```python
from build123d import *

# Parameters (mm, degrees)
RESSALTO_EXTRUS_O1_DEPTH         = 5
ESBO_O2_W                        = 10
ESBO_O2_H                        = 30
ESBO_O2_W_2                      = 30
ESBO_O2_H_2                      = 8
CORTE_EXTRUS_O1_DEPTH            = 5
RESSALTO_EXTRUS_O2_DEPTH         = 5
FURO_COM_FOLGA_DE_M61_D          = 6.6
FURO_COM_FOLGA_DE_M51_D          = 5.5
CORTE_EXTRUS_O2_DEPTH            = 427.059799089
ESBO_O9_W                        = 4
ESBO_O9_H                        = 100
CORTE_EXTRUS_O3_DEPTH            = 417.461117513
FURO_COM_FOLGA_DE_M52_AT_2_COUNT = 2
FURO_COM_FOLGA_DE_M52_AT_2_PITCH = 36.977943225
FURO_COM_FOLGA_DE_M52_AT_3_COUNT = 2
FURO_COM_FOLGA_DE_M52_AT_3_PITCH = 73.955886449


with BuildPart() as part:
    # Esboço1 → Ressalto-extrusão1 (new body)
    with BuildSketch(Plane.XY):
        Polygon((230, 172.82), (360, 172.82), (360, 0), (0, 0), (0, 172.82), (130, 172.82), (130, 134.82), (230, 134.82), align=None)
    extrude(amount=RESSALTO_EXTRUS_O1_DEPTH)

    # Esboço2 → Corte-extrusão1 (cut)
    with BuildSketch(Plane.XY.offset(5)):
        with Locations((5, 61.5)):
            Rectangle(ESBO_O2_W, ESBO_O2_H)
        with Locations((355, 61.5)):
            Rectangle(ESBO_O2_W, ESBO_O2_H)
        with Locations((180, 4)):
            Rectangle(ESBO_O2_W_2, ESBO_O2_H_2)
    extrude(amount=-CORTE_EXTRUS_O1_DEPTH, mode=Mode.SUBTRACT)

    # Esboço3 → Ressalto-extrusão2 (add)
    with BuildSketch(Plane.XY.offset(5)):
        Polygon((360, 172.82), (360, 187.82), (250, 227.82), (250, 172.82), align=None)
        Polygon((0, 187.82), (110, 227.82), (110, 172.82), (0, 172.82), align=None)
    extrude(amount=-RESSALTO_EXTRUS_O2_DEPTH)

    # Furo com folga de M61 (through all)
    with Locations(Plane(origin=(0, 0, 0), x_dir=(-1, 0, 0), z_dir=(0, 0, -1))):
        with Locations((-355, 24.65), (-355, 86.5), (-5, 24.65), (-5, 86.5), (-320, 128.82), (-290, 128.82), (-70, 128.82), (-40, 128.82), (-177, 128.82), (-355, 101.5), (-5, 101.5), (-260, 128.82), (-100, 128.82), (-152, 128.82)):
            Hole(FURO_COM_FOLGA_DE_M61_D / 2)

    # Furo com folga de M51 (through all)
    with Locations(Plane(origin=(0, 0, 0), x_dir=(-1, 0, 0), z_dir=(0, 0, -1))):
        with Locations((-312, 17), (-312, 52.5), (-306.78, 4), (-207.78, 4), (-152.22, 4), (-53.22, 4)):
            furo_com_folga_de_m51 = Hole(FURO_COM_FOLGA_DE_M51_D / 2)

    # Espelhar1: Furo com folga de M51 across plane
    add(furo_com_folga_de_m51.mirror(Plane(origin=(180, 0, 0), x_dir=(0, 0, 1), z_dir=(1, 0, 0))), mode=Mode.SUBTRACT)

    # Esboço8 → Corte-extrusão2 (cut, through all)
    with BuildSketch(Plane.XY.offset(5)):
        Polygon((0, 187.82), (110, 227.82), (110, 209.32), (0, 171.82), align=None)
        Polygon((250, 209.32), (360, 171.82), (360, 187.82), (250, 227.82), align=None)
    extrude(amount=-CORTE_EXTRUS_O2_DEPTH, mode=Mode.SUBTRACT)

    # Esboço9 → Corte-extrusão3 (cut, through all)
    with BuildSketch(Plane.XY.offset(5)):
        with Locations((108, 222.82)):
            Rectangle(ESBO_O9_W, ESBO_O9_H)
        with Locations((252, 222.82)):
            Rectangle(ESBO_O9_W, ESBO_O9_H)
    extrude(amount=-CORTE_EXTRUS_O3_DEPTH, mode=Mode.SUBTRACT)

    # Esboço11 → Furo com folga de M52 (revolve, cut)
    with BuildSketch(Plane(origin=(91, 198.616676618, 5), x_dir=(0, -1, 0), z_dir=(1, 0, 0))):
        Polygon((0, 0), (0, 16.59228064), (2.65, 15), (2.65, 0), align=None)
    furo_com_folga_de_m52 = revolve(axis=Axis((91, 198.616676618, 11.35), (0, 0, -1)), mode=Mode.SUBTRACT)

    # Furo com folga de M52 at 2: Furo com folga de M52 ×2
    with Locations(*[Vector(-0.94651018817854, -0.3226739277881387, 0) * (i * FURO_COM_FOLGA_DE_M52_AT_2_PITCH) for i in range(1, FURO_COM_FOLGA_DE_M52_AT_2_COUNT)]):
        add(furo_com_folga_de_m52, mode=Mode.SUBTRACT)

    # Furo com folga de M52 at 3: Furo com folga de M52 ×2
    with Locations(*[Vector(-0.9465101881785398, -0.322673927788139, 0) * (i * FURO_COM_FOLGA_DE_M52_AT_3_PITCH) for i in range(1, FURO_COM_FOLGA_DE_M52_AT_3_COUNT)]):
        add(furo_com_folga_de_m52, mode=Mode.SUBTRACT)

    # Espelhar2: Furo com folga de M52 across plane
    add(furo_com_folga_de_m52.mirror(Plane(origin=(180, 0, 0), x_dir=(0, 0, 1), z_dir=(1, 0, 0))), mode=Mode.SUBTRACT)

    # Espelhar2 copy 1 sketch → Espelhar2 copy 1 (revolve, cut)
    with BuildSketch(Plane(origin=(304, 186.684858437, 5), x_dir=(0, -1, 0), z_dir=(-1, 0, 0))):
        Polygon((0, 0), (0, -16.59228064), (2.65, -15), (2.65, 0), align=None)
    revolve(axis=Axis((304, 186.684858437, 11.35), (0, 0, 1)), mode=Mode.SUBTRACT)

    # Espelhar2 copy 2 sketch → Espelhar2 copy 2 (revolve, cut)
    with BuildSketch(Plane(origin=(339, 174.753040255, 5), x_dir=(0, -1, 0), z_dir=(-1, 0, 0))):
        Polygon((0, 0), (0, -16.59228064), (2.65, -15), (2.65, 0), align=None)
    revolve(axis=Axis((339, 174.753040255, 11.35), (0, 0, 1)), mode=Mode.SUBTRACT)


solid = part.part
```
Design review of the part built by this model. Coordinates are the model's own, in mm. Give positions to 0.01 mm unless a question says otherwise; leave off trailing zeros. Order: outer loops, then holes, each group sorted by start corner. A loop starts at its lowest first (then second) coordinate and runs counter-clockwise, first axis right, second up. Notation, with made-up numbers: (83, 89) -> (117, 89) arc R16 cw to (117, 119) -> close; hole circle Ø5 at (31, -37.75). An arc over 180 degrees is marked (long way). Write item = value, one per line. Start each with the question number.
(1) We need section D-D on x = 144. Write out the cut boundary in (y, z), plus the area to 3 significant figures.
(2) We need section B-B on z = 3.5. State how many separate pieces and enclosed holes the cut face has, plus the area to 3 significant figures.
(3) To check wall thickness, follow line 1 along Y through (x, z) = (152.22, 3.95); line 2 along X through (y, z) = (23, 1.65); line 3 along Y through (x, z) = (5, 1.3). State the ranges of each line that lie inside material, in increasing order.
(4) For pin 1 (1.5 mm diameter, centred on x = 181, z = 4.5, fed in from -Y); pin 2 (6 mm diameter, centred on x = 5, y = 24.65, fed in from -Z); pin 3 (2 mm diameter, centred on y = 57.5, z = 3.5, fed in from -X), all flat-tipped, find the tip position at first contact; note any pin that passes through.
(5) We need section C-C on x = 332.5. Write out the cut boundary in (y, z) (3 decimals).
(6) We need section A-A on y = 160.5. Write out the cut boundary in (x, z).
(7) Mouldability with a two-part tool opening along X and no side actions: class faces 1 (the face through (177, 82, 0)), 2 (the face through (53.74, 190.14, 2.54)), 3 (the face through (174.57, 131.05, 2.54)) as +X half, -X half, draft (parallel to the pull), parting line (faces both ways), or undercut.
Numbers:
q1.outline = (0, 0) -> (134.82, 0) -> (134.82, 5) -> (0, 5) -> close
q1.area = 674 mm^2
q2.separate_pieces = 1
q2.enclosed_holes = 28
q2.area = 60,400 mm^2
q3.line_1 = 0 to 1.25, 6.75 to 125.53, 132.11 to 134.82
q3.line_2 = 0 to 2.14, 7.86 to 352.14, 357.86 to 360
q3.line_3 = 0 to 21.35, 27.95 to 46.5, 76.5 to 83.2, 89.8 to 98.2, 104.8 to 173.52
q4.pin_1 = 8
q4.pin_2 = through
q4.pin_3 = 10
q5.outline = (0, 0) -> (181.195, 0) -> (181.195, 5) -> (0, 5) -> close
q6.outline = (0, 0) -> (130, 0) -> (130, 5) -> (0, 5) -> close; (230, 0) -> (360, 0) -> (360, 5) -> (230, 5) -> close
q7.face_1 = draft
q7.face_2 = -X half
q7.face_3 = undercut
